Geometry check sheet. Reference: the model listing, model coordinates, mm. A direction names the side the tool comes from. Give positions to 0.01 mm unless a question says otherwise; leave off trailing zeros. Write each loop counter-clockwise with the first axis right and the second up, starting at its lowest first coordinate (ties: lowest second). Pieces come first, ordered by that corner, then holes. Notation, with made-up numbers: (48.25, -23) -> (65.25, -23) arc R21 cw to (65.25, -7) -> close; hole circle Ø3 at (-5, 63.5). An arc over 180 degrees is marked (long way). One line per item, written item: value.
from build123d import *

# Parameters (mm, degrees)
F0_W     = 18
F0_H     = 114
F1_DEPTH = 52
F2_W     = 17
F2_H     = 112
F3_DEPTH = 51
F4_W     = 18
F4_H     = 15
F4_R     = 1
F5_DEPTH = 1
F6_W     = 70
F6_H     = 4
F7_DEPTH = 1
F8_W     = 10
F8_H     = 10
F9_DEPTH = 11.2


with BuildPart() as f1:
    # F0 (on Top) → F1 (new body)
    with BuildSketch(Plane.XY):
        with Locations((-9, 0)):
            Rectangle(F0_W, F0_H)
    extrude(amount=F1_DEPTH)

    # F2 (on face) → F3 (cut)
    with BuildSketch(Plane(origin=(0, 0, 0), x_dir=(1, 0, 0), z_dir=(0, 0, -1))):
        with Locations((-8.5, 0)):
            Rectangle(F2_W, F2_H)
    extrude(amount=-F3_DEPTH, mode=Mode.SUBTRACT)

    # F4 (on Top) → F5 (join)
    with BuildSketch(Plane.XY):
        with Locations((-9, 64.5)):
            Rectangle(F4_W, F4_H)
        with Locations((-9, 64.5)):
            Circle(F4_R, mode=Mode.SUBTRACT)
        with Locations((-9, -64.5)):
            Rectangle(F4_W, F4_H)
        with Locations((-9, -64.5)):
            Circle(F4_R, mode=Mode.SUBTRACT)
    extrude(amount=F5_DEPTH)

    # F6 (on face) → F7 (cut)
    with BuildSketch(Plane.YZ.offset(-17)):
        with Locations((11, 20)):
            Rectangle(F6_W, F6_H)
    extrude(amount=-F7_DEPTH, mode=Mode.SUBTRACT)

    # F8 (on face) → F9 (join)
    with BuildSketch(Plane.YZ.offset(-17)):
        with Locations((-48, 46)):
            Rectangle(F8_W, F8_H)
        with Locations((51, 46)):
            Rectangle(F8_W, F8_H)
    extrude(amount=F9_DEPTH)


solid = f1.part
1) Sectioned sample at D-D on z = 48.5. Record the cut outline in (x, y), plus the area to 3 significant figures.
Verdict:
outline: (-18, -57) -> (0, -57) -> (0, -56) -> (-17, -56) -> (-17, -53) -> (-5.8, -53) -> (-5.8, -43) -> (-17, -43) -> (-17, 46) -> (-5.8, 46) -> (-5.8, 56) -> (0, 56) -> (0, 57) -> (-18, 57) -> close
area: 372 mm^2
2) Tool access check on faces 4 (the flat face through (-9, 1, 52)), 5 (the flat face through (-9, -66, 1)), 6 (the flat face through (-9, 57, 26)), 7 (the flat face through (-5.8, -48, 46)). Record the directions out of +Z, -Z, +X, -X, +Y, -Y that give a thin tool (end or side, any length) a straight path to the whole face; none if there is none.
Verdict:
face 4: +Z, +X, -X, +Y, -Y
face 5: +Z, +X, -X, -Y
face 6: +Z, +X, -X, +Y
face 7: -Z, +X
3) Sectioned sample at A-A on y = -10.5. Record the cut outline in (x, z).
Verdict:
outline: (-18, 0) -> (-17, 0) -> (-17, 18) -> (-18, 18) -> close; (-18, 22) -> (-17, 22) -> (-17, 51) -> (0, 51) -> (0, 52) -> (-18, 52) -> close
4) Sectioned sample at B-B on z = 28. Record the cut outline in (x, y), plus the area to 3 significant figures.
Verdict:
outline: (-18, -57) -> (0, -57) -> (0, -56) -> (-17, -56) -> (-17, 56) -> (0, 56) -> (0, 57) -> (-18, 57) -> close
area: 148 mm^2
5) Sectioned sample at C-C on x = -15.75. Record the cut outline in (y, z), plus the area to 3 significant figures.
Verdict:
outline: (-72, 0) -> (-56, 0) -> (-56, 51) -> (-53, 51) -> (-53, 41) -> (-43, 41) -> (-43, 51) -> (46, 51) -> (46, 41) -> (56, 41) -> (56, 0) -> (72, 0) -> (72, 1) -> (57, 1) -> (57, 52) -> (-57, 52) -> (-57, 1) -> (-72, 1) -> close
area: 446 mm^2
6) Depth check by flat-ended pin: pin 1 Ø9 at (x, z) = (-11.5, 21.5) entering from +Y; pin 2 Ø5 at (y, z) = (23, 22.5) entering from +X; pin 3 Ø5 at (x, z) = (-15, 32.5) entering from -Y. Enter the tip coordinate at first touch or a pass-through.
Verdict:
pin 1: y = 57
pin 2: x = -17
pin 3: y = -57
7) Mould release check, pull along Y, two halves, no side actions. Record for faces 1 (the flat face through (-9, 63, 1)), 2 (the flat face through (-5.8, 51, 46)), 3 (the flat face through (-9, -57, 26)): released by +Y, released by -Y, zero draft, split by the parting line, or undercut.
Verdict:
face 1: zero draft
face 2: undercut
face 3: released by -Y
8) Scan lines: probe 1 along Y at (x, z) = (-9, 0.3); probe 2 along Y at (x, z) = (-11.75, 42); probe 3 along X at (y, z) = (-64.5, 0.65). Record each from-to range of solid material in increasing order.
Verdict:
probe 1: -72 to -65.5, -63.5 to -56, 56 to 63.5, 65.5 to 72
probe 2: -57 to -56, -53 to -43, 46 to 57
probe 3: -18 to -10, -8 to 0
